Verification items for the finished model (mm, model axes). A direction names the side the tool comes from. Give positions to 0.01 mm unless a question says otherwise; leave off trailing zeros. Order: outer loops, then holes, each group sorted by start corner. A loop starts at its lowest first (then second) coordinate and runs counter-clockwise, first axis right, second up.
(1) Sectioned sample at D-D on y = 35.5. Record the cut outline in (x, z), plus the area to 3 significant figures.
(2) Scan lines: L1, parallel to X at y = 44.5, z = -12; L2, parallel to Y at x = -5, z = 0; L3, parallel to X at y = 56.5, z = 0. Record each from-to range of solid material in increasing order.
(3) Sectioned sample at A-A on z = 12. Record the cut outline in (x, y), plus the area to 3 significant figures.
(4) Sectioned sample at C-C on y = 10. Record the cut outline in (x, z).
(5) Sectioned sample at B-B on x = -20.5. Record the cut outline in (y, z), plus the area to 3 significant figures.
(6) Gauge pin test, flat ends, axial feed: pin 1 (17 mm diameter, centred on y = 42.5, z = -4.5, fed in from -X); pin 2 (2.5 mm diameter, centred on x = -20, z = 4.5, fed in from -Y); pin 3 (3.5 mm diameter, centred on x = -32, z = 4, fed in from -Y); pin 4 (4 mm diameter, centred on y = 8.5, z = 1.5, fed in from +X). Record the tip position at first contact, or that the pin passes through.
(7) Mould release check, pull along Z, two halves, no side actions. Record for faces 1 (the face through (-1, 40, -17)), 2 (the face through (-5.5, 34, 0)), 3 (the face through (-0.424, 25.859, -0.189)): pulls with the +Z half, pulls with the -Z half, needs draft (parallel to the pull), parting line crosses it, or undercut.
(8) Access from +Z, -Z, +X, -X, +Y, -Y to the whole of each face (thin tool, end or side, straight path). Record for faces 4 (the face through (1.13, 27.2, -0.19)), 5 (the face through (-17, 64, 0)), 6 (the face through (-18, 54.4, 0)).
```python
from build123d import *

# Parameters (mm, degrees)
SKETCH2_W           = 11
SKETCH2_H           = 34
BOSS_EXTRUDE1_DEPTH = 67
SKETCH3_W           = 34
SKETCH3_H           = 12
BOSS_EXTRUDE2_DEPTH = 30
SKETCH10_W          = 8
SKETCH10_H          = 0.6
SKETCH10_W_2        = 0.6
SKETCH10_H_2        = 8
BOSS_EXTRUDE3_DEPTH = 34
CUT_SWEEP1_START    = -13.5
CUT_SWEEP1_DEPTH    = 27
FILLET1_R           = 4
SKETCH7_R           = 2.25
CUT_EXTRUDE1_DEPTH  = 78.706177469
SKETCH8_R           = 2.25
CUT_EXTRUDE2_DEPTH  = 81.367904146
CHAMFER1_SIZE       = 3
CHAMFER2_SIZE       = 1
SKETCH9_R           = 3.5
CUT_EXTRUDE3_DEPTH  = 6
SKETCH11_R          = 4
CUT_EXTRUDE4_DEPTH  = 5


# Read off the part's stored shape, not the designer's step: Cut-Sweep1
with BuildPart() as part:
    # Sketch2 → Boss-Extrude1 (new body)
    with BuildSketch(Plane(origin=(0, 0, 0), x_dir=(1, 0, 0), z_dir=(0, 1, 0))):
        Rectangle(SKETCH2_W, SKETCH2_H)
    extrude(amount=BOSS_EXTRUDE1_DEPTH)

    # Sketch3 → Boss-Extrude2 (add)
    with BuildSketch(Plane.ZY.offset(5.5)):
        with Locations((0, 61)):
            Rectangle(SKETCH3_W, SKETCH3_H)
    extrude(amount=BOSS_EXTRUDE2_DEPTH)

    # Sketch10 → Boss-Extrude3 (add)
    with BuildSketch(Plane.XY.offset(17)):
        with Locations((-20.5, 54.7)):
            Rectangle(SKETCH10_W, SKETCH10_H)
        with Locations((-5.8, 10)):
            Rectangle(SKETCH10_W_2, SKETCH10_H_2)
    extrude(amount=-BOSS_EXTRUDE3_DEPTH)

    # Cut-Sweep1 outline → Cut-Sweep1 (cut)
    with BuildSketch(Plane.XY.offset(CUT_SWEEP1_START)):
        with BuildLine():
            ThreePointArc((5.5, 22), (1.083592135, 27.291796068), (-0.5, 34))
            Line((-0.5, 34), (-0.5, 56))
            ThreePointArc((-0.5, 56), (1.257359313, 60.242640687), (5.5, 62))
            Line((5.5, 62), (5.5, 64))
            ThreePointArc((5.5, 64), (-0.156854249, 61.656854249), (-2.5, 56))
            Line((-2.5, 56), (-2.5, 34))
            ThreePointArc((-2.5, 34), (-0.366068747, 25.753788749), (5.5, 19.577794898))
            Line((5.5, 19.577794898), (5.5, 22))
        make_face()
    extrude(amount=CUT_SWEEP1_DEPTH, mode=Mode.SUBTRACT)

    # Fillet1
    # the kernel refuses this fillet: 4 mm, written as the material it takes off along each edge
    with BuildSketch(Plane(origin=(5.5, -10, 17), x_dir=(0, 0, -1), z_dir=(0, 1, 0))) as fillet1_piece_1:
        with BuildLine():
            CenterArc((FILLET1_R, FILLET1_R), FILLET1_R, 180, 90)
            Line((0, FILLET1_R), (0, 0))
            Line((0, 0), (FILLET1_R, 0))
        make_face()
    extrude(amount=87, mode=Mode.SUBTRACT)

    # Sketch7 → Cut-Extrude1 (cut, through all)
    with BuildSketch(Plane(origin=(0, 67, 0), x_dir=(1, 0, 0), z_dir=(0, 1, 0))):
        with Locations(Location((-20.5, 0, 0), (0, 0, 270))):
            Circle(SKETCH7_R)
    extrude(amount=-CUT_EXTRUDE1_DEPTH, mode=Mode.SUBTRACT)

    # Sketch8 → Cut-Extrude2 (cut, through all)
    with BuildSketch(Plane(origin=(5.5, 0, 0), x_dir=(0, 0, -1), z_dir=(1, 0, 0))):
        with Locations((0, 10)):
            Circle(SKETCH8_R)
    extrude(amount=-CUT_EXTRUDE2_DEPTH, mode=Mode.SUBTRACT)

    # Chamfer1
    chamfer1_edges = [part.edges().sort_by_distance(p)[0] for p in [
        (-2, 0, 17),
        (5.5, 0, -2),
        (4.328427125, 0, 15.828427125),
    ]]
    chamfer(chamfer1_edges, length=CHAMFER1_SIZE)

    # Chamfer2
    chamfer2_edges = [part.edges().sort_by_distance(p)[0] for p in [
        (-17, 67, 17),
        (5.5, 67, -2),
        (4.328427125, 67, 15.828427125),
    ]]
    chamfer(chamfer2_edges, length=CHAMFER2_SIZE)

    # Sketch9 → Cut-Extrude3 (cut)
    with BuildSketch(Plane(origin=(0, 67, 0), x_dir=(1, 0, 0), z_dir=(0, 1, 0))):
        with Locations(Location((-20.5, 0, 0), (0, 0, 270))):
            Circle(SKETCH9_R)
    extrude(amount=-CUT_EXTRUDE3_DEPTH, mode=Mode.SUBTRACT)

    # Sketch11 → Cut-Extrude4 (cut)
    with BuildSketch(Plane(origin=(5.5, 0, 0), x_dir=(0, 0, -1), z_dir=(1, 0, 0))):
        with Locations((0, 10)):
            Circle(SKETCH11_R)
    extrude(amount=-CUT_EXTRUDE4_DEPTH, mode=Mode.SUBTRACT)


solid = part.part
```
Ans:
1. outline: (-5.5, -17) - (5.5, -17) - (5.5, 13) arc R4 ccw to (1.5, 17) - (-5.5, 17) - close; hole (-2.5, -13.5) - (-0.5, -13.5) - (-0.5, 13.5) - (-2.5, 13.5) - close
1. area: 317 mm2
2. L1: x = -5.5 to -2.5, -0.5 to 5.5
2. L2: y = 0 to 7.75, 12.25 to 67
2. L3: x = -35.5 to -22.75, -18.25 to -2.48, -0.48 to 5.5
3. outline: (-35.5, 55) - (-24.5, 55) - (-24.5, 54.4) - (-16.5, 54.4) - (-16.5, 55) - (-5.5, 55) - (-5.5, 14) - (-6.1, 14) - (-6.1, 6) - (-5.5, 6) - (-5.5, 0) - (2.5, 0) - (5.5, 3) - (5.5, 19.58) arc R17 cw to (-2.5, 34) - (-2.5, 56) arc R8 cw to (5.5, 64) - (5.5, 66) - (4.5, 67) - (-35.5, 67) - close; (-0.5, 34) arc R15 ccw to (5.5, 22) - (5.5, 62) arc R6 ccw to (-0.5, 56) - close
3. area: 1,000 mm2
4. outline: (-6.1, -17) - (5.5, -17) - (5.5, -4) - (0.5, -4) - (0.5, -2.25) - (-6.1, -2.25) - close; (-6.1, 2.25) - (0.5, 2.25) - (0.5, 4) - (5.5, 4) - (5.5, 13) arc R4 ccw to (1.5, 17) - (-6.1, 17) - close
5. outline: (54.4, -17) - (67, -17) - (67, -3.5) - (61, -3.5) - (61, -2.25) - (54.4, -2.25) - close; (54.4, 2.25) - (61, 2.25) - (61, 3.5) - (67, 3.5) - (67, 16) - (66, 17) - (54.4, 17) - close
5. area: 356 mm2
6. pin 1: stops at x = -5.5
6. pin 2: stops at y = 54.4
6. pin 3: stops at y = 55
6. pin 4: stops at x = 5.5
7. face 1: pulls with the -Z half
7. face 2: needs draft
7. face 3: undercut
8. face 4: none
8. face 5: +Y
8. face 6: +Z, -Z, -X, -Y
